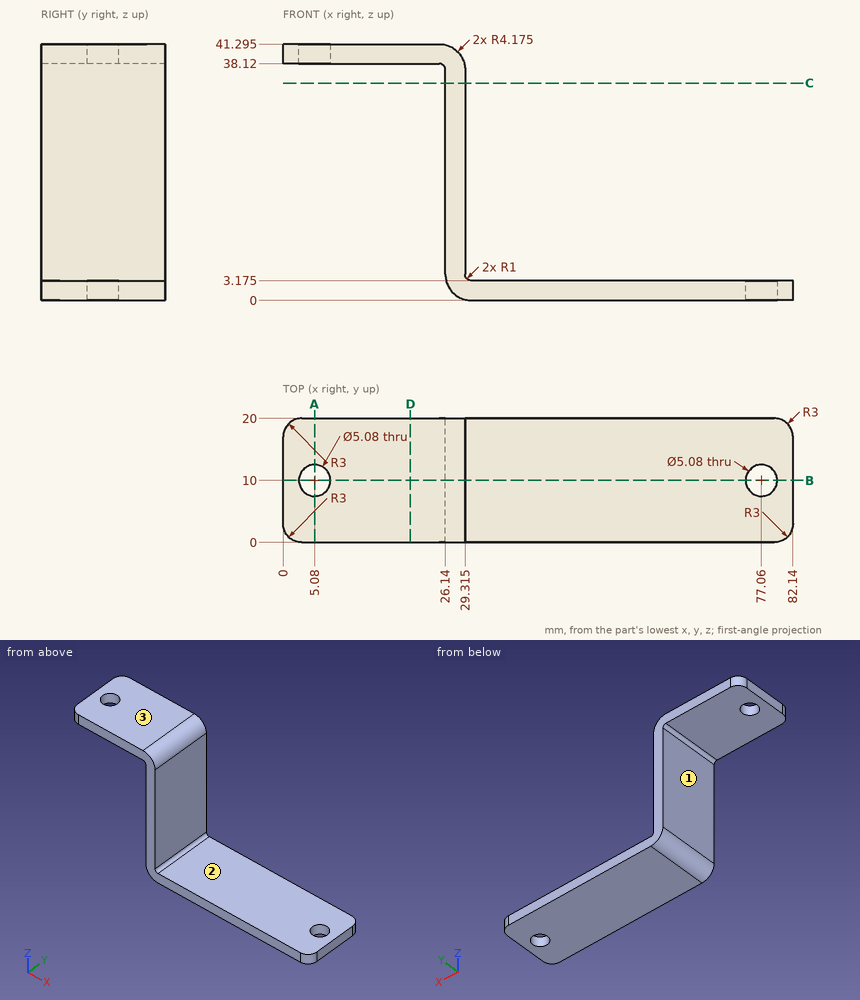
For this review, use the dimensioned drawing (mm, ordinates from the lowest corner) and the shaded views. A direction names the side the tool comes from. Give positions to 0.01 mm unless a question says otherwise; leave off trailing zeros. Order: outer loops, then holes, each group sorted by start corner. A loop starts at its lowest first (then second) coordinate and runs counter-clockwise, first axis right, second up.
1. Add section B-B, the plane y = 10. State how many separate pieces and enclosed holes the cut face has.
Solution:
separate pieces: 3
enclosed holes: 0
2. Add section A-A, the plane x = 5.08. State the section outline as (y, z) points (1 decimal).
Solution:
outline: (0, 38.1) - (7.5, 38.1) - (7.5, 41.3) - (0, 41.3) - close; (12.5, 38.1) - (20, 38.1) - (20, 41.3) - (12.5, 41.3) - close
3. To check wall thickness, follow L1, parallel to Y at x = 5, z = 40; L2, parallel to X at y = 19, z = 21 (1 decimal); L3, parallel to X at y = 10, z = 1.8. State the ranges of each line that lie inside material, in increasing order.
Solution:
L1: y = 0 to 7.46, 12.54 to 20
L2: x = 26.1 to 29.3
L3: x = 26.88 to 74.52, 79.6 to 82.14
4. Add section C-C, the plane z = 35. State the section outline as (x, y) points (1 decimal).
Solution:
outline: (26.1, 0) - (29.3, 0) - (29.3, 20) - (26.1, 20) - close
5. Add section D-D, the plane x = 20.5. State the section outline as (y, z) points (1 decimal), then the cut area to 3 significant figures.
Solution:
outline: (0, 38.1) - (20, 38.1) - (20, 41.3) - (0, 41.3) - close
area: 63.5 mm2
6. Tool access review of the marked faces 1, 2 and 3: name each direction out of +Z, -Z, +X, -X, +Y, -Y from which nothing blocks a thin tool from reaching the whole face with its end or side.
Solution:
face 1: -Z, -X, +Y, -Y
face 2: +Z, +X, +Y, -Y
face 3: +Z, +X, -X, +Y, -Y
7. For pin 1 Ø1.5 at (x, y) = (70, 6) entering from +Z (3 decimals); pin 2 Ø4 at (x, y) = (5.08, 10) entering from -Z; pin 3 Ø8 at (y, z) = (7.5, 28.5) entering from -X; pin 4 Ø10 at (x, y) = (32, 14) entering from +Z, all flat-tipped, find the tip position at first contact; note any pin that passes through.
Solution:
pin 1: stops at z = 3.175
pin 2: passes through
pin 3: stops at x = 26.14
pin 4: stops at z = 40.86
